Input: part model. Units: mm. Frame: model coordinates. Coordinates: 2 decimals unless noted, no trailing zeros. Write each loop counter-clockwise with the first axis right and the second up, starting at its lowest first coordinate (ties: lowest second). Pieces come first, ordered by that corner, then holes. Notation, with made-up numbers: (-30, 47.25) - (-15, 47.25) arc R25 cw to (-15, 82.25) - close; hole circle Ø4 at (-6.75, 36.25). An arc over 180 degrees is marked (long way). Use CSV: the item, a comma, the result in double quotes.
```python
from build123d import *

# Parameters (mm, degrees)
SKETCH_1_R      = 2.25
SKETCH_1_R_2    = 4.25
EXTRUDE_1_DEPTH = 11


with BuildPart() as part:
    # 草图1 → 凸台-拉伸1 (new body)
    with BuildSketch(Plane.XY):
        with BuildLine():
            Line((-56.82826087, 9.961271461), (43.17173913, 9.961271461))
            Line((43.17173913, 9.961271461), (43.17173913, -15.038728539))
            Line((43.17173913, -15.038728539), (-56.82826087, -15.038728539))
            ThreePointArc((-56.82826087, -15.038728539), (-69.32826087, -2.538728539), (-56.82826087, 9.961271461))
        make_face()
        with Locations((33.17173913, -2.538728539)):
            Circle(SKETCH_1_R, mode=Mode.SUBTRACT)
        with Locations((24.17173913, -2.538728539)):
            Circle(SKETCH_1_R, mode=Mode.SUBTRACT)
        with Locations((8.17173913, -2.538728539)):
            Circle(SKETCH_1_R, mode=Mode.SUBTRACT)
        with Locations((-56.82826087, -2.538728539)):
            Circle(SKETCH_1_R_2, mode=Mode.SUBTRACT)
    extrude(amount=EXTRUDE_1_DEPTH)


solid = part.part
```
(1) Cut plane B-B on z = 3.5. Return loops of the section in (x, y).
Check values:
outline,"(-56.83, -15.04) - (43.17, -15.04) - (43.17, 9.96) - (-56.83, 9.96) arc R12.5 ccw to start; hole circle Ø8.5 at (-56.83, -2.54); hole circle Ø4.5 at (8.17, -2.54); hole circle Ø4.5 at (24.17, -2.54); hole circle Ø4.5 at (33.17, -2.54)"
(2) Cut plane D-D on y = 5.25. Return loops of the section in (x, z).
Check values:
outline,"(-66.61, 0) - (43.17, 0) - (43.17, 11) - (-66.61, 11) - close"
(3) Draft query along Y for faces 1 (the flat face through (-12, -2, 0)), 2 (the cylindrical face through (-69.325, -2.814, 5.423)), 3 (the cylindrical face through (6.39, -3.91, 5.42)). Return one class per face: pulls with the +Y half, pulls with the -Y half, needs draft (parallel to the pull), parting line crosses it, or undercut.
Check values:
face 1,"needs draft"
face 2,"parting line crosses it"
face 3,"undercut"
(4) Ray query, probe 1 along Y at (x, z) = (33, 8.5); probe 2 along X at (y, z) = (-4.5, 10.5); probe 3 along X at (y, z) = (-3.75, 4.5). Return the intervals inside material, ascending. Write a range as from..to.
Check values:
probe 1,"-15.04..-4.78, -0.3..9.96"
probe 2,"-69.17..-60.6, -53.06..7.07, 9.27..23.07, 25.27..32.07, 34.27..43.17"
probe 3,"-69.27..-60.9, -52.75..6.28, 10.07..22.28, 26.07..31.28, 35.07..43.17"
(5) Cut plane C-C on x = 24.5. Return loops of the section in (y, z), and give its area (3 significant figures).
Check values:
outline,"(-15.04, 0) - (-4.76, 0) - (-4.76, 11) - (-15.04, 11) - close; (-0.31, 0) - (9.96, 0) - (9.96, 11) - (-0.31, 11) - close"
area,"226 mm^2"
(6) Cut plane A-A on y = -1.5. Return loops of the section in (x, z).
Check values:
outline,"(-69.29, 0) - (-60.95, 0) - (-60.95, 11) - (-69.29, 11) - close; (-52.71, 0) - (6.18, 0) - (6.18, 11) - (-52.71, 11) - close; (10.17, 0) - (22.18, 0) - (22.18, 11) - (10.17, 11) - close; (26.17, 0) - (31.18, 0) - (31.18, 11) - (26.17, 11) - close; (35.17, 0) - (43.17, 0) - (43.17, 11) - (35.17, 11) - close"
(7) Pin query (flat end, axial travel): pin 1 Ø4 at (x, y) = (33.17, -2.54) entering from +Z; pin 2 Ø3 at (y, z) = (-10.5, 7) entering from -X; pin 3 Ø2 at (y, z) = (-0.5, 6) entering from -X (3 decimals). Return the tip coordinate at first contact, or that it passes through.
Check values:
pin 1,"through"
pin 2,"x = -67.53"
pin 3,"x = -69.285"
